```python
from build123d import *

# Parameters (mm, degrees)
BASPROSKE_W           = 15
BASPROSKE_H           = 39.5
TOOTHCUT_DEPTH        = 213.661703181
TEETHCUTS_COUNT       = 36
TEETHCUTS_ANGLE       = 350
CROQUIS1_OUTSIDE_W    = 386.906
CROQUIS1_OUTSIDE_H    = 386.906
CROQUIS1_OUTSIDE_W_2  = 205.376556513
CROQUIS1_OUTSIDE_H_2  = 174.679952659
CORTAR_EXTRUIR1_DEPTH = 213.661703181
CROQUIS2_R            = 2
CORTAR_EXTRUIR2_DEPTH = 213.661703181
CROQUIS2_3_R          = 3
CROQUIS2_3_R_2        = 2
CORTAR_EXTRUIR3_DEPTH = 3


with BuildPart() as part:
    # BasProSke → Base-Revolve (revolve)
    with BuildSketch(Plane(origin=(0, 0, 0), x_dir=(1, 0, 0), z_dir=(0, 1, 0)), mode=Mode.PRIVATE) as base_revolve_sk:
        with Locations((7.5, 130.25)):
            Rectangle(BASPROSKE_W, BASPROSKE_H)
    revolve(base_revolve_sk.sketch.rotate(Axis((-10, 0, 0), (1, 0, 0)), 180), axis=Axis((-10, 0, 0), (1, 0, 0)))

    # TooCutSke → ToothCut (cut, through all)
    with BuildSketch(Plane(origin=(0, 0, 0), x_dir=(0, 0, -1), z_dir=(1, 0, 0))):
        with BuildLine():
            ThreePointArc((7.872935628, 110.193711843), (5.234019781, 117.874768587), (1.556724153, 125.116315826))
            ThreePointArc((1.556724153, 125.116315826), (0, 125.126), (-1.556724153, 125.116315826))
            ThreePointArc((-1.556724153, 125.116315826), (-5.234019781, 117.874768587), (-7.872935628, 110.193711843))
            ThreePointArc((-7.872935628, 110.193711843), (0, 110.4746), (7.872935628, 110.193711843))
        make_face()
    toothcut = extrude(amount=TOOTHCUT_DEPTH, mode=Mode.SUBTRACT)

    # TeethCuts: ToothCut ×36 about axis
    teethcuts_axis = Axis((-10, 0, 0), (1, 0, 0))
    for i in range(1, TEETHCUTS_COUNT):
        add(toothcut.rotate(teethcuts_axis, i * TEETHCUTS_ANGLE / (TEETHCUTS_COUNT - 1)), mode=Mode.SUBTRACT)

    # Croquis1 outside → Cortar-Extruir1 (cut, through all)
    with BuildSketch(Plane(origin=(15, 0, 0), x_dir=(0, 0, -1), z_dir=(1, 0, 0))):
        Rectangle(CROQUIS1_OUTSIDE_W, CROQUIS1_OUTSIDE_H)
        with Locations((-102.688278257, 87.33997633)):
            Rectangle(CROQUIS1_OUTSIDE_W_2, CROQUIS1_OUTSIDE_H_2, mode=Mode.SUBTRACT)
    extrude(amount=-CORTAR_EXTRUIR1_DEPTH, mode=Mode.SUBTRACT)

    # Croquis2 → Cortar-Extruir2 (cut, through all)
    with BuildSketch(Plane(origin=(15, 0, 0), x_dir=(0, 0, -1), z_dir=(1, 0, 0))):
        with Locations((-23.963448518, 135.903469916)):
            Circle(CROQUIS2_R)
        with Locations((-99.268892447, 95.862855123)):
            Circle(CROQUIS2_R)
        with Locations((-136.656993486, 19.205887932)):
            Circle(CROQUIS2_R)
    extrude(amount=-CORTAR_EXTRUIR2_DEPTH, mode=Mode.SUBTRACT)

    # Croquis2_3 → Cortar-Extruir3 (cut)
    # profile 1 of 3: a face of its own
    with BuildSketch(Plane(origin=(15, 0, 0), x_dir=(0, 0, -1), z_dir=(1, 0, 0))):
        with Locations((-136.656993486, 19.205887932)):
            Circle(CROQUIS2_3_R)
        with Locations((-136.656993486, 19.205887932)):
            Circle(CROQUIS2_3_R_2, mode=Mode.SUBTRACT)
    # profile 2 of 3: a face of its own
    with BuildSketch(Plane(origin=(15, 0, 0), x_dir=(0, 0, -1), z_dir=(1, 0, 0))):
        with Locations((-99.268892447, 95.862855123)):
            Circle(CROQUIS2_3_R)
        with Locations((-99.268892447, 95.862855123)):
            Circle(CROQUIS2_3_R_2, mode=Mode.SUBTRACT)
    # profile 3 of 3: a face of its own
    with BuildSketch(Plane(origin=(15, 0, 0), x_dir=(0, 0, -1), z_dir=(1, 0, 0))):
        with Locations((-23.963448518, 135.903469916)):
            Circle(CROQUIS2_3_R)
        with Locations((-23.963448518, 135.903469916)):
            Circle(CROQUIS2_3_R_2, mode=Mode.SUBTRACT)
    extrude(amount=-CORTAR_EXTRUIR3_DEPTH, mode=Mode.SUBTRACT)


solid = part.part
```
The model under review builds one solid part; all positions refer to its coordinate system, in mm. A direction names the side the tool comes from. Give positions to 0.01 mm unless a question says otherwise; leave off trailing zeros. Write each loop counter-clockwise with the first axis right and the second up, starting at its lowest first coordinate (ties: lowest second). Pieces come first, ordered by that corner, then holes. Notation, with made-up numbers: M 22.25,53 L 60.25,53 A22 ccw 60.25,64 Z; hole C 79,86 d10. An arc over 180 degrees is marked long. Answer in a Markdown table with one row per item.
Item 1: Add section A-A on y = 104. Give the boundary of the cut face in (x, z), plus the area to 3 significant figures.
Check sheet entries:
| item | result |
|---|---|
| outline | M 0,45.28 L 15,45.28 L 15,53.5 L 0,53.5 Z; M 0,63.85 L 15,63.85 L 15,108.09 L 0,108.09 Z |
| area | 787 mm2 |
Item 2: For P1, Ø8, axis at x = 10, z = 31, coming from the -Y side; P2, Ø6, axis at x = 10.5, y = 27, coming from the +Z side; P3, Ø5, axis at y = 135.9, z = 23.96, coming from the +X side; P4, Ø4.5, axis at y = 95.86, z = 99.27, coming from the -X side, all flat-tipped, find the tip position at first contact; note any pin that passes through.
Check sheet entries:
| item | result |
|---|---|
| P1 | y = 106.26 |
| P2 | z = 148.07 |
| P3 | x = 12 |
| P4 | x = 0 |
Item 3: For line 1 along Z through (x, y) = (1.75, 114.5); line 2 along Z through (x, y) = (3.75, 106); line 3 along Y through (x, z) = (2.25, 94), list the stretches that pass through material, from the lowest coordinate up.
Check sheet entries:
| item | result |
|---|---|
| line 1 | 6.54 to 13.79, 25.77 to 37.29, 44.69 to 96.9 |
| line 2 | 45.31 to 56.2, 63.91 to 106.13 |
| line 3 | 62.53 to 72.43, 81.47 to 116.89 |
Item 4: Add section D-D on z = 33. Give the boundary of the cut face in (x, y).
Check sheet entries:
| item | result |
|---|---|
| outline | M 0,109.81 L 15,109.81 L 15,146.32 L 0,146.32 Z |
Item 5: Add section C-C on y = 121. Give the boundary of the cut face in (x, z), plus the area to 3 significant figures.
Check sheet entries:
| item | result |
|---|---|
| outline | M 0,3.8 L 15,3.8 L 15,18.16 L 0,18.16 Z; M 0,23.96 L 15,23.96 L 15,88.65 L 0,88.65 Z |
| area | 1,190 mm2 |
Item 6: Draft analysis for pull direction Y (two halves, no side actions). For faces 5 (the face through (7.395, 104.639, 54.325)), 6 (the face through (7.6, 107.23, 104.89)), 7 (the face through (7.4, 63.46, 99.37)), state which applies: +Y half, -Y half, draft (parallel to the pull), parting line (faces both ways), or undercut.
Check sheet entries:
| item | result |
|---|---|
| face 5 | -Y half |
| face 6 | +Y half |
| face 7 | undercut |
Item 7: Tool access review of faces 1 (the face through (7.4, 116.91, 15.26)), 2 (the face through (13.521, 18.057, 133.886)), 3 (the face through (7.395, 5.273, 117.782)), 4 (the face through (7.4, 79.75, 86.84)): name each direction out of +Z, -Z, +X, -X, +Y, -Y from which nothing blocks a thin tool from reaching the whole face with its end or side.
Check sheet entries:
| item | result |
|---|---|
| face 1 | +X, -X, -Y |
| face 2 | +X |
| face 3 | -Z, +X, -X, -Y |
| face 4 | +X, -X |
Item 8: Add section B-B on z = 136.5. Give the boundary of the cut face in (x, y).
Check sheet entries:
| item | result |
|---|---|
| outline | M 0,0 L 15,0 L 15,16.21 L 12,16.21 L 12,17.21 L 0,17.21 Z; M 0,21.2 L 12,21.2 L 12,22.2 L 15,22.2 L 15,62.19 L 0,62.19 Z |
